Read the model definition and answer for the solid it produces. Units are mm, in the model's axes. Round coordinates to 2 decimals unless told otherwise and drop trailing zeros. Order: outer loops, then holes, each group sorted by start corner. A loop starts at its lowest first (then second) coordinate and runs counter-clockwise, first axis right, second up. Notation, with made-up numbers: (42.5, -36.5) -> (85.5, -36.5) arc R23 ccw to (85.5, -25.5) -> close; hole circle Ø4 at (-12.5, -28.5). An arc over 180 degrees is marked (long way). Use a Markdown table: item, result. Add a question column.
1. Given pin 1 (2 mm diameter, centred on y = 2, z = 74, fed in from +X); pin 2 (5 mm diameter, centred on x = -20.5, z = 243, fed in from -Y); pin 3 (2 mm diameter, centred on y = 0.5, z = 104, fed in from +X); pin 4 (1.2 mm diameter, centred on y = 2.5, z = 19.5, fed in from -X), each flat-ended and moving along its own axis, determine where each tip first touches the part or whether it passes through.
2. Section A-A, the plane y = 0.6 is taken. Give the number of separate pieces and of enclosed holes in the cut face, then the cut area to 3 significant figures.
3. The mould has two halves that part along Y. Classify faces 1 (the face through (-64.35, 1.972, 314.263)), 2 (the face through (1, 4, 156)), 3 (the face through (1, 0, 156)): +Y half, -Y half, draft (parallel to the pull), parting line (faces both ways), or undercut.
4. Consider L1, parallel to Z at x = -28.9, y = 0.8; L2, parallel to X at y = 3.2, z = 225.5; L3, parallel to Z at x = 33.1, y = 2.5. Determine where each line is inside the solid, lowest interval first. Write a range as [from, to].
5. Section B-B, the plane z = 294 is taken. Give the vertices of the cut face in (x, y), then the cut area to 3 significant figures.
```python
from build123d import *

# Parameters (mm, degrees)
BOSS_EXTRUDE1_DEPTH                        = 4
F_3_3_3_3_GATEN_TANDWIELKAST_D             = 3.3
F_2_5_2_5_BATTERIJ_HOUDER_D                = 2.5
F_2_7_2_7_ARDUINO_GATEN_D2_7_D             = 2.7
F_3_2_3_2_ARDUINO_GATEN_D3_2_D             = 3.2
F_3_2_3_2_BREADBOARD_ONDERSTEUNINGSPLAAT_D = 3.2


with BuildPart() as part:
    # grondplaat groene golf → Boss-Extrude1 (new body)
    with BuildSketch(Plane(origin=(0, 0, 0), x_dir=(1, 0, 0), z_dir=(0, 1, 0))):
        with BuildLine():
            Line((-55, 0), (55, 0))
            ThreePointArc((55, 0), (59.949747468, -2.050252532), (62, -7))
            Line((62, -7), (62, -30))
            Line((62, -30), (28, -30))
            Line((28, -30), (28, -90))
            Line((28, -90), (62, -90))
            Line((62, -90), (70, -220))
            Line((70, -220), (25, -220))
            Line((25, -220), (25, -280))
            Line((25, -280), (70, -280))
            Line((70, -280), (66.691886591, -309.773020683))
            ThreePointArc((66.691886591, -309.773020683), (64.403150685, -314.215896125), (59.734700448, -316))
            Line((59.734700448, -316), (-59.734700448, -316))
            ThreePointArc((-59.734700448, -316), (-64.403150685, -314.215896125), (-66.691886591, -309.773020683))
            Line((-66.691886591, -309.773020683), (-70, -280))
            Line((-70, -280), (-25, -280))
            Line((-25, -280), (-25, -220))
            Line((-25, -220), (-70, -220))
            Line((-70, -220), (-62, -90))
            Line((-62, -90), (-28, -90))
            Line((-28, -90), (-28, -30))
            Line((-28, -30), (-62, -30))
            Line((-62, -30), (-62, -7))
            ThreePointArc((-62, -7), (-59.949747468, -2.050252532), (-55, 0))
        make_face()
    extrude(amount=BOSS_EXTRUDE1_DEPTH)

    # Ø3.3 (3.3) gaten tandwielkast (through all)
    with Locations(Plane(origin=(0, 4, 0), x_dir=(1, 0, 0), z_dir=(0, 1, 0))):
        with Locations((11.5, -278.5), (-0.5, -278.5), (-0.5, -225.5), (11.5, -225.5)):
            Hole(F_3_3_3_3_GATEN_TANDWIELKAST_D / 2)

    # Ø2.5 (2.5) batterij houder (through all)
    with Locations(Plane(origin=(0, 4, 0), x_dir=(1, 0, 0), z_dir=(0, 1, 0))):
        with Locations((-55, -205), (-32.8, -191), (-55, -177)):
            Hole(F_2_5_2_5_BATTERIJ_HOUDER_D / 2)

    # Ø2.7 (2.7) Arduino gaten D2.7 (through all)
    with Locations(Plane(origin=(0, 4, 0), x_dir=(1, 0, 0), z_dir=(0, 1, 0))):
        with Locations((-39, -105.09), (-39, -133), (11.76, -148.23), (13.03, -100.01)):
            Hole(F_2_7_2_7_ARDUINO_GATEN_D2_7_D / 2)

    # Ø3.2 (3.2) Arduino gaten D3.2 (through all)
    with Locations(Plane(origin=(0, 4, 0), x_dir=(1, 0, 0), z_dir=(0, 1, 0))):
        with Locations((-28.9, -104.87), (-28.9, -143.37), (33.1, -99.62), (33.1, -148.62)):
            Hole(F_3_2_3_2_ARDUINO_GATEN_D3_2_D / 2)

    # Ø3.2 (3.2) Breadboard ondersteuningsplaatje (through all)
    with Locations(Plane(origin=(0, 4, 0), x_dir=(1, 0, 0), z_dir=(0, 1, 0))):
        with Locations((-5, -160), (60, -160), (-5, -215), (60, -215)):
            Hole(F_3_2_3_2_BREADBOARD_ONDERSTEUNINGSPLAAT_D / 2)


solid = part.part
```
Verdict:
| question | item | result |
|---|---|---|
| 1 | pin 1 | stops at x = 28 |
| 1 | pin 2 | stops at y = 0 |
| 1 | pin 3 | stops at x = 62.92 |
| 1 | pin 4 | stops at x = -62 |
| 2 | separate pieces | 1 |
| 2 | enclosed holes | 19 |
| 2 | area | 32,000 mm2 |
| 3 | face 1 | draft |
| 3 | face 2 | +Y half |
| 3 | face 3 | -Y half |
| 4 | L1 | z = [0, 30], [90, 103.27], [106.47, 141.77], [144.97, 220], [280, 316] |
| 4 | L2 | x = [-25, -2.15], [1.15, 9.85], [13.15, 25] |
| 4 | L3 | z = [0, 30], [90, 98.02], [101.22, 147.02], [150.22, 220], [280, 316] |
| 5 | outline | (-68.44, 0) -> (68.44, 0) -> (68.44, 4) -> (-68.44, 4) -> close |
| 5 | area | 548 mm2 |
